Design review of the part shown in the three views and the two pictorial views. Dimensions are in mm from the part's minimum x, y and z. Coordinates: 2 decimals unless noted, no trailing zeros. Answer as CSV lines item,"result". Start each with the question number.
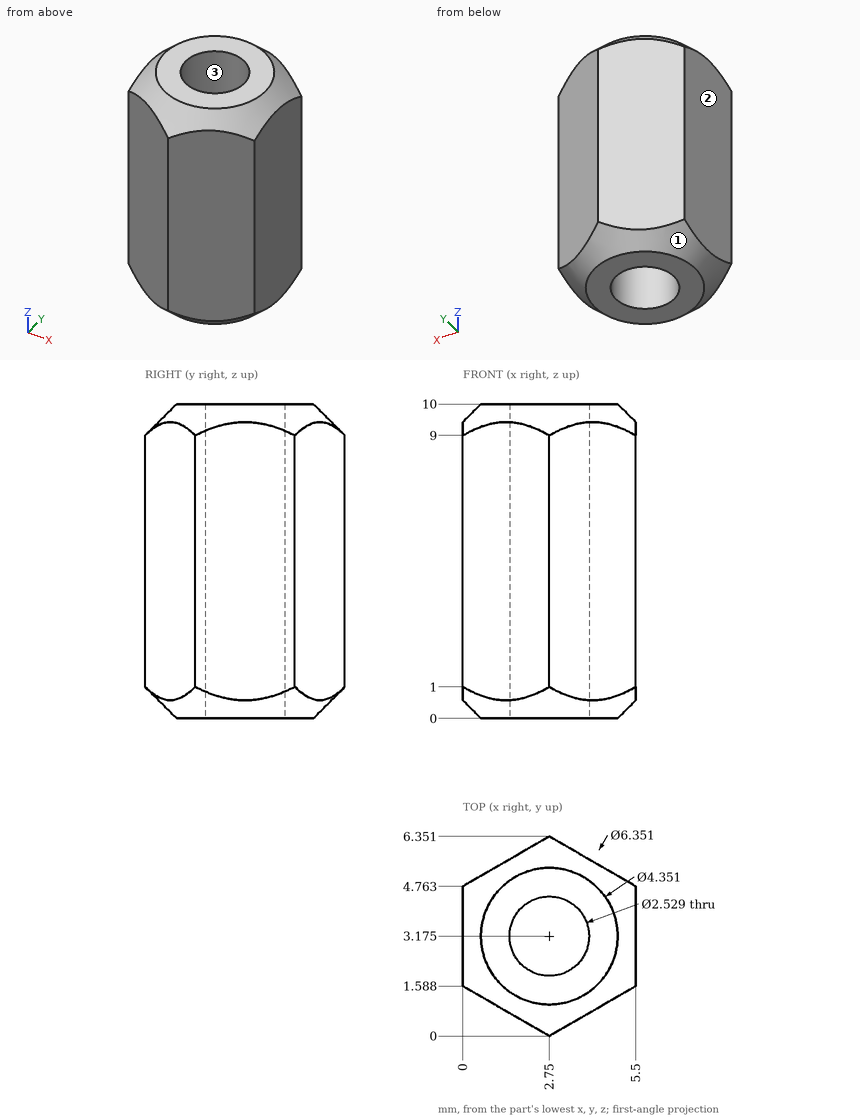
1) Insertion check: pin 1 Ø2 at (x, y) = (2.75, 3.18) entering from -Z; pin 2 Ø1 at (x, z) = (1, 5.5) entering from +Y; pin 3 Ø3 at (x, z) = (3.5, 3.5) entering from -Y. Each pin has a flat end and moves straight along its axis. Give the tip position at first contact, or say it passes through.
2) Wall thickness on L1, parallel to X at y = 3.25, z = 5.75; L2, parallel to X at y = 2.5, z = 5; L3, parallel to Y at x = 3.45, z = 6 (1 decimal): over which ranges is each line inside the solid? List them lowest first. Write a range as [from, to].
3) Mouldability with a two-part tool opening along X and no side actions: class the marked faces 1, 2 and 3 as released by +X, released by -X, zero draft, split by the parting line, or undercut.
Result:
1,pin 1,"through"
1,pin 2,"y = 5.63"
1,pin 3,"y = 0"
2,L1,"[0, 1.49], [4.01, 5.5]"
2,L2,"[0, 1.68], [3.82, 5.5]"
2,L3,"[0.4, 2.1], [4.2, 5.9]"
3,face 1,"split by the parting line"
3,face 2,"released by -X"
3,face 3,"undercut"
